```python
from build123d import *

# Parameters (mm, degrees)
F0_W     = 6.35
F0_H     = 50.8
F2_ANGLE = 30
F3_W     = 6.35
F3_H     = 12.7
F4_ANGLE = 20
F5_ANGLE = 10
F6_R     = 1.27
F7_R     = 1.11125
F9_R     = 0.254


with BuildPart() as f2:
    # F0 (on Right) → F2 (revolve)
    with BuildSketch(Plane.YZ):
        with Locations((-47.625, 25.4)):
            Rectangle(F0_W, F0_H)
    revolve(axis=Axis((0, 0, 29.2990189046), (0, 0, 1)), revolution_arc=F2_ANGLE)

    # F3 (on Right) → F4 (revolve)
    with BuildSketch(Plane.YZ):
        with Locations((-47.625, 57.15)):
            Rectangle(F3_W, F3_H)
    revolve(axis=Axis((0, 0, 29.2990189046), (0, 0, 1)), revolution_arc=F4_ANGLE)

    # F3 (on Right) → F5 (revolve, cut)
    with BuildSketch(Plane.YZ):
        with Locations((-47.625, 57.15)):
            Rectangle(F3_W, F3_H)
    revolve(axis=Axis((0, 0, 29.2990189046), (0, 0, 1)), revolution_arc=F5_ANGLE, mode=Mode.SUBTRACT)

    # F6
    f6_edges = [f2.edges().sort_by_distance(p)[0] for p in [
        (16.288709, -44.752861, 63.5),
        (8.269994, -46.901469, 63.5),
        (23.8125, -41.24446, 50.8),
        (8.269994, -46.901469, 50.8),
        (0, -47.625, 0),
        (23.8125, -41.24446, 0),
        (16.288709, -44.752861, 50.8),
        (0, -47.625, 50.8),
    ]]
    fillet(f6_edges, radius=F6_R)

    # F7 (on Right) → F8 (revolve, cut)
    with BuildSketch(Plane.YZ):
        with Locations((-47.625, 38.1)):
            Circle(F7_R)
        with Locations((-47.625, 12.7)):
            Circle(F7_R)
    revolve(axis=Axis((0, 0, 29.2990189046), (0, 0, 1)), mode=Mode.SUBTRACT)

    # F9
    f9_edges = [f2.edges().sort_by_distance(p)[0] for p in [
        (24.368125, -42.206831, 38.1),
        (24.368125, -42.206831, 12.7),
        (0, -48.73625, 38.1),
        (0, -48.73625, 12.7),
    ]]
    fillet(f9_edges, radius=F9_R)


solid = f2.part
```
Read the model definition and answer for the solid it produces. Units are mm, in the model's axes. A direction names the side the tool comes from. Round coordinates to 2 decimals unless told otherwise and drop trailing zeros. Write each loop counter-clockwise with the first axis right and the second up, starting at its lowest first coordinate (ties: lowest second). Pieces come first, ordered by that corner, then holes. Notation, with made-up numbers: (40.25, -20) -> (80.25, -20) arc R14 cw to (80.25, -12) -> close; hole circle Ø2 at (25.5, 26.5). An arc over 180 degrees is marked (long way). Answer in a Markdown table with one row per item. Add a question column.
1) Consider line 1 (Z direction, x = 21.5, y = -45.5); line 2 (Y direction, x = 20.75, z = 38); line 3 (Y direction, x = 1.5, z = 21). Determine where each line is inside the solid, lowest interval first.
2) Given P1, Ø3, axis at x = 4.5, y = -48, coming from the +Z side; P2, Ø2, axis at y = -42, z = 21, coming from the +X side, each flat-ended and moving along its own axis, determine where each tip first touches the part or whether it passes through.
3) Find section D-D, the plane z = 55. Determine the outline of the cut face in (x, y).
4) Find section B-B, the plane x = 12. State how many separate pieces and enclosed holes the cut face has, and give its area (3 significant figures).
5) Which of the six approach directions +Z, -Z, +X, -X, +Y, -Y give full straight-line access (tool end or side, diameter ignored) to faces 1 (the face through (8.28, -46.95, 57.22)), 2 (the face through (12.968, -49.117, 25.139)), 3 (the face through (16.304, -44.795, 57.221))?
6) Find section A-A, the plane z = 18. Determine the outline of the cut face in (x, y) (3 decimals).
Findings below:
| question | item | result |
|---|---|---|
| 1 | line 1 | 0 to 50.8 |
| 1 | line 2 | -46.37 to -44.09, -41.63 to -39.31 |
| 1 | line 3 | -50.78 to -44.42 |
| 2 | P1 | z = 50.8 |
| 2 | P2 | x = 24.83 |
| 3 | outline | (7.72, -43.77) -> (8.82, -50.03) arc R50.8 ccw to (17.37, -47.74) -> (15.2, -41.77) arc R44.45 cw to start |
| 4 | separate pieces | 1 |
| 4 | enclosed holes | 2 |
| 4 | area | 409 mm² |
| 5 | face 1 | +Z, -X, -Y |
| 5 | face 2 | +Z, -Z, +X, -Y |
| 5 | face 3 | +Z, +X, +Y |
| 6 | outline | (0, -50.8) arc R50.8 ccw to (25.4, -43.994) -> (22.225, -38.495) arc R44.45 cw to (0, -44.45) -> close |
